Verification items for the finished model (mm, model axes). A direction names the side the tool comes from. Coordinates: 2 decimals unless noted, no trailing zeros. Order: outer loops, then holes, each group sorted by start corner. A loop starts at its lowest first (then second) coordinate and runs counter-clockwise, first axis right, second up.
Q1. Cross-section at C-C, the plane x = 121. Record the boundary of the cut face in (y, z).
Q2. Draft check along Z on faces 5 (the flat face through (179, 0, -140)), 6 (the flat face through (130, 31, 0)), 7 (the flat face through (75, 5, -140)). Enter one of: pulls with the +Z half, pulls with the -Z half, needs draft (parallel to the pull), parting line crosses it, or undercut.
Q3. Set-up check for faces 1 (the flat face through (19, 31, -300)), 2 (the flat face through (243, 7, -300)), 3 (the flat face through (261.9, 19, -300)), 4 (the flat face through (75, 33.1, -140)): record each of +Z, -Z, +X, -X, +Y, -Y from which the full face is reachable in a straight line by a thin tool's end or side.
Q4. Cross-section at D-D, the plane z = -18. Record the boundary of the cut face in (x, y).
Q5. Depth check by flat-ended pin: P1, Ø7, axis at x = 146, y = 6, coming from the +Z side; P2, Ø11, axis at x = 237, y = 7, coming from the -Z side; P3, Ø19, axis at x = 125.5, y = 21.5, coming from the -Z side. Enter the tip coordinate at first touch or a pass-through.
Q6. Cross-section at A-A, the plane z = -77. Record the boundary of the cut face in (x, y), and give its area (3 significant figures).
Q7. Thickness scan on line 1 (X direction, y = 17, z = -55); line 2 (X direction, y = 11, z = -271); line 3 (Y direction, x = 36, z = -270). Record the ranges inside material, lowest first.
Q8. Cross-section at B-B, the plane y = 19.05. Record the boundary of the cut face in (x, z), and give its area (3 significant figures).
from build123d import *

# Parameters (mm, degrees)
BOSS_EXTRUDE1_DEPTH = 38.1
SWEEP1_PROFILE_R    = 5
SWEEP2_PROFILE_R    = 5
SWEEP4_PROFILE_R    = 5
SHELL4_START        = 5
SHELL4_DEPTH        = 28.1


# Read off the part's stored shape, not the designer's step: Shell4
with BuildPart() as part:
    # Sketch1 → Boss-Extrude1 (new body)
    with BuildSketch(Plane(origin=(0, 0, 0), x_dir=(1, 0, 0), z_dir=(0, 1, 0))):
        Polygon((111.9, 0), (150, 0), (177.363917526, 0), (261.9, 300), (223.8, 300), (150, 38.1), (111.9, 38.1), (38.1, 300), (0, 300), (84.536082474, 0), align=None)
    extrude(amount=BOSS_EXTRUDE1_DEPTH)

    # Sweep1: sweep along a path in Sketch2
    with BuildLine(Plane.XY) as sweep1_path:
        Line((84.536082474, 19.05), (177.363917526, 19.05))
    # Sweep1 profile (on start of the path) → Sweep1 (sweep)
    with BuildSketch(Plane(origin=(84.536082474, 19.05, 0), x_dir=(0, 0, 1), z_dir=(1, 0, 0))):
        Circle(SWEEP1_PROFILE_R)
    sweep(path=sweep1_path.line)

    # Sweep2: sweep along a path in Sketch11
    with BuildLine(Plane(origin=(0, 0, -300), x_dir=(-1, 0, 0), z_dir=(0, 0, -1))) as sweep2_path:
        Line((0, 19.05), (-38.1, 19.05))
    # Sweep2 profile (on start of the path) → Sweep2 (sweep)
    with BuildSketch(Plane(origin=(0, 19.05, -300), x_dir=(0, 0, 1), z_dir=(1, 0, 0))):
        Circle(SWEEP2_PROFILE_R)
    sweep(path=sweep2_path.line)

    # Sweep4: sweep along a path in Sketch16
    with BuildLine(Plane(origin=(0, 0, -300), x_dir=(-1, 0, 0), z_dir=(0, 0, -1))) as sweep4_path:
        Line((-261.9, 19.05), (-223.8, 19.05))
    # Sweep4 profile (on start of the path) → Sweep4 (sweep)
    with BuildSketch(Plane(origin=(261.9, 19.05, -300), x_dir=(0, 0, -1), z_dir=(-1, 0, 0))):
        Circle(SWEEP4_PROFILE_R)
    sweep(path=sweep4_path.line)

    # Shell4 outline → Shell4 (cut)
    with BuildSketch(Plane(origin=(0, 0, 0), x_dir=(1, 0, 0), z_dir=(0, 1, 0)).offset(SHELL4_START)):
        Polygon((255.296347108, 295), (227.585783476, 295), (153.785783476, 33.1), (108.114216524, 33.1), (34.314216524, 295), (6.603652892, 295), (88.32186595, 5), (173.57813405, 5), align=None)
    extrude(amount=SHELL4_DEPTH, mode=Mode.SUBTRACT)


solid = part.part
Check values:
1. outline: (0, -38.1) - (38.1, -38.1) - (38.1, 0) - (24.05, 0) arc R5 ccw to (14.05, 0) - (0, 0) - close; hole (5, -33.1) - (33.1, -33.1) - (33.1, -5) - (5, -5) - close
2. face 5: needs draft
2. face 6: pulls with the +Z half
2. face 7: undercut
3. face 1: -Z, +X, -X, +Y
3. face 2: -Z, +X, -X, -Y
3. face 3: +Z, -Z, +X, +Y, -Y
3. face 4: none
4. outline: (79.46, 0) - (182.44, 0) - (182.44, 38.1) - (79.46, 38.1) - close; hole (84.66, 5) - (177.24, 5) - (177.24, 33.1) - (84.66, 33.1) - close
5. P1: stops at z = 0
5. P2: stops at z = -300
5. P3: stops at z = -38.1
6. outline: (62.84, 0) - (100.94, 0) - (100.94, 38.1) - (62.84, 38.1) - close; (160.96, 0) - (199.06, 0) - (199.06, 38.1) - (160.96, 38.1) - close; hole (68.03, 5) - (95.74, 5) - (95.74, 33.1) - (68.03, 33.1) - close; hole (166.16, 5) - (193.87, 5) - (193.87, 33.1) - (166.16, 33.1) - close
6. area: 1,350 mm2
7. line 1: x = 69.04 to 74.23, 101.94 to 107.14, 154.76 to 159.96, 187.67 to 192.86
7. line 2: x = 8.17 to 13.37, 41.08 to 46.27, 215.63 to 220.82, 248.53 to 253.73
7. line 3: y = 0 to 5, 33.1 to 38.1
8. outline: (0, -305) - (38.1, -305) - (38.1, -300) - (111.9, -38.1) - (150, -38.1) - (223.8, -300) - (223.8, -305) - (261.9, -305) - (261.9, -295) - (260.49, -295) - (177.36, 0) - (177.36, 5) - (84.54, 5) - (84.54, 0) - (1.41, -295) - (0, -295) - close; hole (6.6, -295) - (34.31, -295) - (108.11, -33.1) - (153.79, -33.1) - (227.59, -295) - (255.3, -295) - (173.58, -5) - (88.32, -5) - close
8. area: 7,620 mm2
